from build123d import *

# Parameters (mm, degrees)
SKETCH1_R           = 2.15
BOSS_EXTRUDE1_DEPTH = 115


with BuildPart() as part:
    # Sketch1 → Boss-Extrude1 (new body)
    with BuildSketch(Plane.XY):
        with BuildLine():
            Line((2, 0), (6.6, 0))
            ThreePointArc((6.6, 0), (7.307106781, 0.292893219), (7.6, 1))
            Line((7.6, 1), (7.6, 2))
            Line((7.6, 2), (5.664213562, 2))
            ThreePointArc((5.664213562, 2), (4.74033403, 2.617316568), (4.957106781, 3.707106781))
            Line((4.957106781, 3.707106781), (7.307106781, 6.057106781))
            ThreePointArc((7.307106781, 6.057106781), (7.63153013, 6.273879533), (8.014213562, 6.35))
            Line((8.014213562, 6.35), (12.185786438, 6.35))
            ThreePointArc((12.185786438, 6.35), (12.56846987, 6.273879533), (12.892893219, 6.057106781))
            Line((12.892893219, 6.057106781), (15.242893219, 3.707106781))
            ThreePointArc((15.242893219, 3.707106781), (15.45966597, 2.617316568), (14.535786438, 2))
            Line((14.535786438, 2), (12.6, 2))
            Line((12.6, 2), (12.6, 1))
            ThreePointArc((12.6, 1), (12.892893219, 0.292893219), (13.6, 0))
            Line((13.6, 0), (18.2, 0))
            ThreePointArc((18.2, 0), (19.614213562, 0.585786438), (20.2, 2))
            Line((20.2, 2), (20.2, 6.6))
            ThreePointArc((20.2, 6.6), (19.907106781, 7.307106781), (19.2, 7.6))
            Line((19.2, 7.6), (18.2, 7.6))
            Line((18.2, 7.6), (18.2, 5.664213562))
            ThreePointArc((18.2, 5.664213562), (17.582683432, 4.74033403), (16.492893219, 4.957106781))
            Line((16.492893219, 4.957106781), (14.142893219, 7.307106781))
            ThreePointArc((14.142893219, 7.307106781), (13.926120467, 7.63153013), (13.85, 8.014213562))
            Line((13.85, 8.014213562), (13.85, 12.185786438))
            ThreePointArc((13.85, 12.185786438), (13.926120467, 12.56846987), (14.142893219, 12.892893219))
            Line((14.142893219, 12.892893219), (16.492893219, 15.242893219))
            ThreePointArc((16.492893219, 15.242893219), (17.582683432, 15.45966597), (18.2, 14.535786438))
            Line((18.2, 14.535786438), (18.2, 12.6))
            Line((18.2, 12.6), (19.2, 12.6))
            ThreePointArc((19.2, 12.6), (19.907106781, 12.892893219), (20.2, 13.6))
            Line((20.2, 13.6), (20.2, 18.2))
            ThreePointArc((20.2, 18.2), (19.614213562, 19.614213562), (18.2, 20.2))
            Line((18.2, 20.2), (13.6, 20.2))
            ThreePointArc((13.6, 20.2), (12.892893219, 19.907106781), (12.6, 19.2))
            Line((12.6, 19.2), (12.6, 18.2))
            Line((12.6, 18.2), (14.535786438, 18.2))
            ThreePointArc((14.535786438, 18.2), (15.45966597, 17.582683432), (15.242893219, 16.492893219))
            Line((15.242893219, 16.492893219), (12.892893219, 14.142893219))
            ThreePointArc((12.892893219, 14.142893219), (12.56846987, 13.926120467), (12.185786438, 13.85))
            Line((12.185786438, 13.85), (8.014213562, 13.85))
            ThreePointArc((8.014213562, 13.85), (7.63153013, 13.926120467), (7.307106781, 14.142893219))
            Line((7.307106781, 14.142893219), (4.957106781, 16.492893219))
            ThreePointArc((4.957106781, 16.492893219), (4.74033403, 17.582683432), (5.664213562, 18.2))
            Line((5.664213562, 18.2), (7.6, 18.2))
            Line((7.6, 18.2), (7.6, 19.2))
            ThreePointArc((7.6, 19.2), (7.307106781, 19.907106781), (6.6, 20.2))
            Line((6.6, 20.2), (2, 20.2))
            ThreePointArc((2, 20.2), (0.585786438, 19.614213562), (0, 18.2))
            Line((0, 18.2), (0, 13.6))
            ThreePointArc((0, 13.6), (0.292893219, 12.892893219), (1, 12.6))
            Line((1, 12.6), (2, 12.6))
            Line((2, 12.6), (2, 14.535786438))
            ThreePointArc((2, 14.535786438), (2.617316568, 15.45966597), (3.707106781, 15.242893219))
            Line((3.707106781, 15.242893219), (6.057106781, 12.892893219))
            ThreePointArc((6.057106781, 12.892893219), (6.273879533, 12.56846987), (6.35, 12.185786438))
            Line((6.35, 12.185786438), (6.35, 8.014213562))
            ThreePointArc((6.35, 8.014213562), (6.273879533, 7.63153013), (6.057106781, 7.307106781))
            Line((6.057106781, 7.307106781), (3.707106781, 4.957106781))
            ThreePointArc((3.707106781, 4.957106781), (2.617316568, 4.74033403), (2, 5.664213562))
            Line((2, 5.664213562), (2, 7.6))
            Line((2, 7.6), (1, 7.6))
            ThreePointArc((1, 7.6), (0.292893219, 7.307106781), (0, 6.6))
            Line((0, 6.6), (0, 2))
            ThreePointArc((0, 2), (0.585786438, 0.585786438), (2, 0))
        make_face()
        with Locations((10.1, 10)):
            Circle(SKETCH1_R, mode=Mode.SUBTRACT)
    extrude(amount=BOSS_EXTRUDE1_DEPTH)


solid = part.part
Input: part model. Units: mm. Frame: model coordinates. A direction names the side the tool comes from. Give positions to 0.01 mm unless a question says otherwise; leave off trailing zeros. Order: outer loops, then holes, each group sorted by start corner. A loop starts at its lowest first (then second) coordinate and runs counter-clockwise, first axis right, second up. Notation, with made-up numbers: (3, 69.5) - (7, 69.5) arc R34 cw to (7, 106.5) - close; hole circle Ø5 at (89.25, -37). An arc over 180 degrees is marked (long way). Answer as a JSON object with one key per item and string values. Group by question number.
Q1. Mould query, pull axis X, two halves, no side actions, for faces 1 (the face through (13.85, 10, 57)), 2 (the face through (6.35, 10, 57)), 3 (the face through (11.09, 8.09, 56.7)). Classes: pulls with the +X half, pulls with the -X half, needs draft (parallel to the pull), parting line crosses it, or undercut.
Q2. First-contact query: pin 1 Ø2 at (y, z) = (13.5, 84.5) entering from +X; pin 2 Ø1 at (x, z) = (13, 36.5) entering from -Y (3 decimals); pin 3 Ø2 at (y, z) = (9.5, 43.5) entering from +X; pin 4 Ø3.5 at (x, z) = (10, 38) entering from +Y. Flat tips, straight axial feed; report the tip coordinate or a pass-through.
Q3. Set-up query: faces 4 (the face through (6.12, 4.87, 56.7)), 5 (the face through (10, 13.85, 57)), 6 (the face through (4, 0, 57)). Return all of +Z, -Z, +X, -X, +Y, -Y with unobstructed straight access to the full face (end or side cutting, diameter ignored); none if empty.
Q4. Cut plane B-B, the plane y = 10. Output: boundary loops of the cut face in (x, z).
Q5. Cut plane A-A, the plane x = 10.1. Output: boundary loops of the cut face in (y, z).
Q6. Line query: probe 1 along Y at (x, z) = (10.1, 46); probe 2 along Y at (x, z) = (18.5, 71.5); probe 3 along Y at (x, z) = (5.5, 90). Output: solid intervals per line, ascending.
Results:
{
 "1": {"face 1": "pulls with the +X half", "face 2": "pulls with the -X half", "face 3": "undercut"},
 "2": {"pin 1": "x = 20.2", "pin 2": "y = 0.005", "pin 3": "x = 13.85", "pin 4": "y = 13.85"},
 "3": {"face 4": "+Z, -Z", "face 5": "+Z, -Z, +Y", "face 6": "+Z, -Z, +X, -X, -Y"},
 "4": {"outline": "(6.35, 0) - (7.95, 0) - (7.95, 115) - (6.35, 115) - close; (12.25, 0) - (13.85, 0) - (13.85, 115) - (12.25, 115) - close"},
 "5": {"outline": "(6.35, 0) - (7.85, 0) - (7.85, 115) - (6.35, 115) - close; (12.15, 0) - (13.85, 0) - (13.85, 115) - (12.15, 115) - close"},
 "6": {"probe 1": "6.35 to 7.85, 12.15 to 13.85", "probe 2": "0.02 to 7.6, 12.6 to 20.18", "probe 3": "0 to 2.01, 4.25 to 6.75, 13.45 to 15.95, 18.19 to 20.2"}
}
